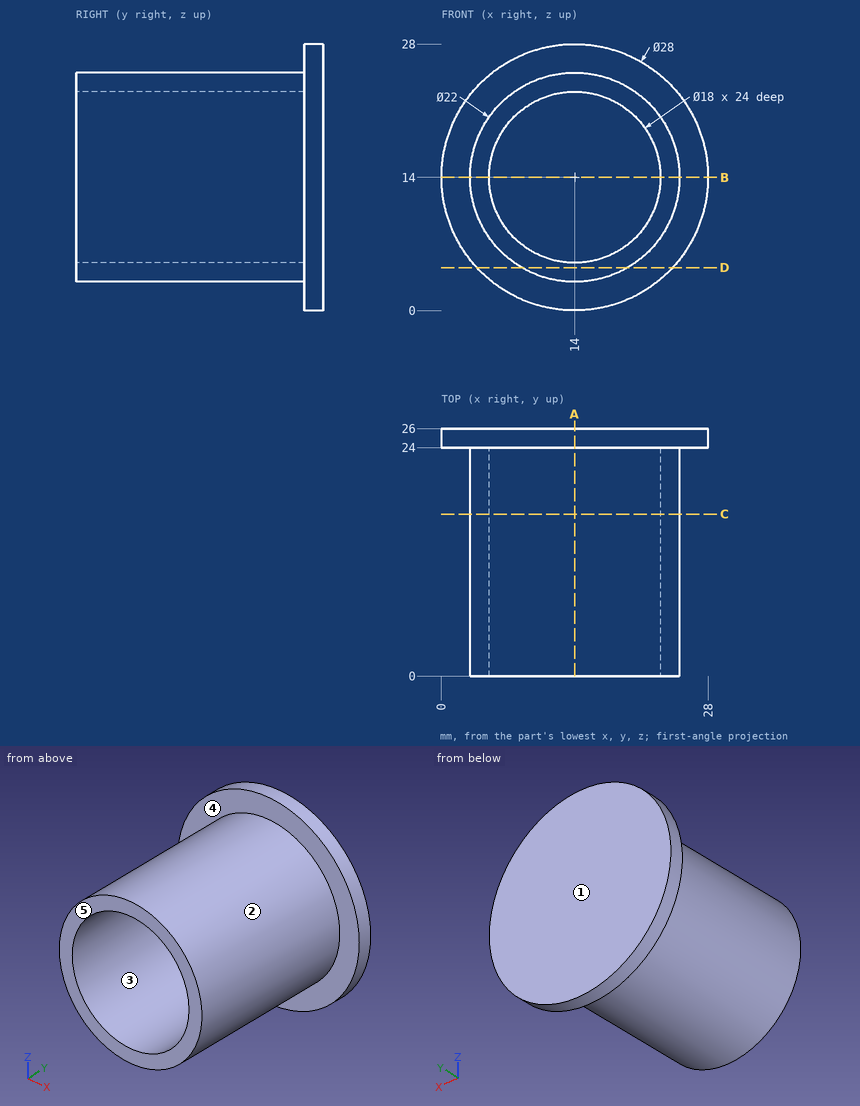
Can you work these out from the drawing? Everything is in mm from the part's minimum corner. A direction names the side the tool comes from. Round coordinates to 2 decimals unless told otherwise and drop trailing zeros. Loops run counter-clockwise (first coordinate to the right, second up) from the corner with the lowest first, then second, coordinate; pieces in that order, holes last. Notation, with made-up numbers: M 49.5,-7.75 L 96.5,-7.75 A18 cw 96.5,8.25 Z; hole C 77,72 d3. An arc over 180 degrees is marked long. Answer in a Markdown table with one row per item.
1. Please list where these lines run through material, in increasing order: line 1 (Z direction, x = 14, y = 7.5); line 2 (Y direction, x = 7.25, z = 3.75); line 3 (X direction, y = 8.75, z = 22). Write a range as from..to.
Established:
| item | result |
|---|---|
| line 1 | 3..5, 23..25 |
| line 2 | 24..26 |
| line 3 | 6.45..9.88, 18.12..21.55 |
2. I'm going to push flat-ended pins straight in: pin 1 Ø5 at (y, z) = (11, 9) entering from +X; pin 2 Ø1 at (x, y) = (19, 18.5) entering from +Z; pin 3 Ø11 at (x, z) = (14, 14) entering from -Y. Where does each tip first touch, or does it pass through?
Established:
| item | result |
|---|---|
| pin 1 | x = 24.71 |
| pin 2 | z = 24.04 |
| pin 3 | y = 24 |
3. If we section it at D-D, the plane z = 4.5: Please give me the cut outline in (x, y).
Established:
| item | result |
|---|---|
| outline | M 3.72,24 L 8.45,24 L 8.45,0 L 19.55,0 L 19.55,24 L 24.28,24 L 24.28,26 L 3.72,26 Z |
4. Thinking about a two-plate mould opening in Z: for the marked faces 1, 2 and 3, which applies, pulls with the +Z half, pulls with the -Z half, needs draft (parallel to the pull), parting line crosses it, or undercut?
Established:
| item | result |
|---|---|
| face 1 | needs draft |
| face 2 | parting line crosses it |
| face 3 | undercut |
5. If we section it at C-C, the plane y = 17: Please give me the cut outline in (x, z).
Established:
| item | result |
|---|---|
| outline | C 14,14 d22; hole C 14,14 d18 |
6. On a 3-axis mill with a long thin cutter (end or side, diameter ignored), from which of +Z, -Z, +X, -X, +Y, -Y can I reach the whole of each face in a straight line? I mean the marked faces 4 and 5. Say none if no direction works.
Established:
| item | result |
|---|---|
| face 4 | -Y |
| face 5 | +Z, -Z, +X, -X, -Y |
7. If we section it at A-A, the plane x = 14: Please give me the cut outline in (y, z).
Established:
| item | result |
|---|---|
| outline | M 0,3 L 24,3 L 24,0 L 26,0 L 26,28 L 24,28 L 24,25 L 0,25 L 0,23 L 24,23 L 24,5 L 0,5 Z |
8. If we section it at B-B, the plane z = 14: Please give me the cut outline in (x, y), plus the area to 3 significant figures.
Established:
| item | result |
|---|---|
| outline | M 0,24 L 3,24 L 3,0 L 5,0 L 5,24 L 23,24 L 23,0 L 25,0 L 25,24 L 28,24 L 28,26 L 0,26 Z |
| area | 152 mm² |
